from build123d import *

# Parameters (mm, degrees)
SKETCH1_R           = 4
BOSS_EXTRUDE1_DEPTH = 10
SKETCH2_W           = 20
SKETCH2_H           = 20
BOSS_EXTRUDE2_DEPTH = 10
SKETCH3_R           = 4
BOSS_EXTRUDE4_DEPTH = 10
FILLET1_R           = 10


with BuildPart() as part:
    # Sketch1 → Boss-Extrude1 (new, symmetric)
    with BuildSketch(Plane.XY):
        with BuildLine():
            Line((-4.683153706, 17.681145748), (-33.683153706, 10))
            Line((-33.683153706, 10), (-33.683153706, -10))
            Line((-33.683153706, -10), (-4.683153706, -17.681145748))
            ThreePointArc((-4.683153706, -17.681145748), (18.290840429, 0), (-4.683153706, 17.681145748))
        make_face()
        Circle(SKETCH1_R, mode=Mode.SUBTRACT)
    extrude(amount=BOSS_EXTRUDE1_DEPTH, both=True)

    # Sketch2 → Boss-Extrude2 (add)
    with BuildSketch(Plane.ZY.offset(33.683153706)):
        Rectangle(SKETCH2_W, SKETCH2_H)
    extrude(amount=BOSS_EXTRUDE2_DEPTH)

    # Sketch3 → Boss-Extrude4 (add, symmetric)
    with BuildSketch(Plane(origin=(0, 0, 0), x_dir=(1, 0, 0), z_dir=(0, 1, 0))):
        with BuildLine():
            Line((-43.683153706, 10), (-72.683153706, 17.681145748))
            ThreePointArc((-72.683153706, 17.681145748), (-95.657147841, 0), (-72.683153706, -17.681145748))
            Line((-72.683153706, -17.681145748), (-43.683153706, -10))
            Line((-43.683153706, -10), (-43.683153706, 10))
        make_face()
        with Locations(Location((-77.366307412, 0, 0), (0, 0, 270))):
            Circle(SKETCH3_R, mode=Mode.SUBTRACT)
    extrude(amount=BOSS_EXTRUDE4_DEPTH, both=True)

    # Fillet1
    fillet1_edges = [part.edges().sort_by_distance(p)[0] for p in [
        (-43.683153706, 0, 10),
        (-43.683153706, 0, -10),
        (-33.683153706, -10, 0),
        (-33.683153706, 10, 0),
    ]]
    fillet(fillet1_edges, radius=FILLET1_R)


solid = part.part
Build history of the part. All positions in model axes, mm. A direction names the side the tool comes from. Give positions to 0.01 mm unless a question says otherwise; leave off trailing zeros. Loops run counter-clockwise (first coordinate to the right, second up) from the corner with the lowest first, then second, coordinate; pieces in that order, holes last. Notation, with made-up numbers: (-33.5, 13) -> (-8.5, 13) arc R19 ccw to (-8.5, 17) -> close; hole circle Ø2 at (50.25, -29). An arc over 180 degrees is marked (long way). Answer in a Markdown table with one row per item.
Item 1: Slice it at C-C on y = 0. Write the cut outline in (x, z).
Findings below:
| item | result |
|---|---|
| outline | (-72.68, -17.68) -> (-44.94, -10.33) arc R10 cw to (-42.38, -10) -> (-4, -10) -> (-4, 10) -> (-42.38, 10) arc R10 cw to (-44.94, 10.33) -> (-72.68, 17.68) arc R18.29 ccw (long way) to start; (4, -10) -> (18.29, -10) -> (18.29, 10) -> (4, 10) -> close; hole circle Ø8 at (-77.37, 0) |
Item 2: Tool access for faces 1 (the flat face through (-66, 10, 0)), 2 (the flat face through (-12, 0, 10)), 3 (the flat face through (-66, -10, 0)), 4 (the flat face through (-12, 0, -10)), 5 (the cylindrical face through (18.285, -0.468, 0.14)): list every direction of +Z, -Z, +X, -X, +Y, -Y with a clear straight run to the whole face (end or side of a thin tool).
Findings below:
| item | result |
|---|---|
| face 1 | +Z, -Z, -X, +Y |
| face 2 | +Z, +X, +Y, -Y |
| face 3 | +Z, -Z, -X, -Y |
| face 4 | -Z, +X, +Y, -Y |
| face 5 | +Z, -Z |
Item 3: Slice it at A-A on z = 0. Write the cut outline in (x, y), plus the area to 3 significant figures.
Findings below:
| item | result |
|---|---|
| outline | (-95.66, -10) -> (-81.37, -10) -> (-81.37, 10) -> (-95.66, 10) -> close; (-73.37, -10) -> (-34.99, -10) arc R10 cw to (-32.42, -10.33) -> (-4.68, -17.68) arc R18.29 ccw (long way) to (-4.68, 17.68) -> (-32.42, 10.33) arc R10 cw to (-34.99, 10) -> (-73.37, 10) -> close; hole circle Ø8 at (0, 0) |
| area | 2,530 mm² |
Item 4: Slice it at B-B on x = 0. Write the cut outline in (y, z).
Findings below:
| item | result |
|---|---|
| outline | (-18.29, -10) -> (-4, -10) -> (-4, 10) -> (-18.29, 10) -> close; (4, -10) -> (18.29, -10) -> (18.29, 10) -> (4, 10) -> close |
Item 5: Slice it at D-D on y = 6. Write the cut outline in (x, z).
Findings below:
| item | result |
|---|---|
| outline | (-72.68, -17.68) -> (-44.94, -10.33) arc R10 cw to (-42.38, -10) -> (17.28, -10) -> (17.28, 10) -> (-42.38, 10) arc R10 cw to (-44.94, 10.33) -> (-72.68, 17.68) arc R18.29 ccw (long way) to start; hole circle Ø8 at (-77.37, 0) |
Item 6: Probe line 1 along Y through (x, z) = (0, 5); line 2 along Y through (x, z) = (-65.5, -2.5); line 3 along Z through (x, y) = (-78.5, 1.5). List the from-to ranges inside material, lowest first. Write a range as [from, to].
Findings below:
| item | result |
|---|---|
| line 1 | y = [-18.29, -4], [4, 18.29] |
| line 2 | y = [-10, 10] |
| line 3 | z = [-18.26, -3.84], [3.84, 18.26] |
Item 7: Flat gauge pins, fed straight in: P1, Ø6, axis at x = -13.5, z = -2.5, coming from the +Y side; P2, Ø12, axis at x = -18.5, z = -2, coming from the -Y side; P3, Ø4, axis at y = 13.5, z = -6.5, coming from the +X side. Where does each tip first touch, or does it go through?
Findings below:
| item | result |
|---|---|
| P1 | stops at y = 16.14 |
| P2 | stops at y = -15.61 |
| P3 | stops at x = 14.22 |
Item 8: Mould opens along Z. For faces 6 (the cylindrical face through (-0.867, -3.905, -0.14)), 7 (the cylindrical face through (-80.915, -0.14, 1.846)), 8 (the cylindrical face through (-95.65, 0.14, -0.47)) say: pulls with the +Z half, pulls with the -Z half, needs draft (parallel to the pull), parting line crosses it, or undercut.
Findings below:
| item | result |
|---|---|
| face 6 | needs draft |
| face 7 | undercut |
| face 8 | parting line crosses it |
